Could you check a few things on this model? Use its own coordinates, in mm. Coordinates: 2 decimals unless noted, no trailing zeros. Write each loop counter-clockwise with the first axis right and the second up, starting at its lowest first coordinate (ties: lowest second). Pieces come first, ordered by that corner, then holes. Notation, with made-up numbers: (78, -20) - (92, -20) arc R15 cw to (92, -4) - close; hole circle Ø10 at (46, -11). An arc over 180 degrees is marked (long way). Write item = value, one per line. Start each with the question number.
```python
from build123d import *

# Parameters (mm, degrees)
F0_R     = 40
F1_DEPTH = 20
F2_R     = 5.08
F3_R     = 5.08


with BuildPart() as f1:
    # F0 (on Top) → F1 (new body)
    with BuildSketch(Plane.XY):
        with BuildLine():
            ThreePointArc((-115.457179, 96.407526), (-144.891009, 9.736149), (-61.108229, 46.597019))
            ThreePointArc((-61.108229, 46.597019), (-74.039839, 80.151967), (-106.145609, 96.350133))
            ThreePointArc((-106.145609, 96.350133), (-110.828783, 91.935219), (-115.457179, 96.407526))
        make_face()
        with Locations((-111.108229, 46.597019)):
            Circle(F0_R, mode=Mode.SUBTRACT)
    extrude(amount=F1_DEPTH)

    # F2
    f2_edges = [f1.edges().sort_by_distance(p)[0] for p in [
        (-151.108229, 46.597019, 20),
    ]]
    fillet(f2_edges, radius=F2_R)

    # F3
    f3_edges = [f1.edges().sort_by_distance(p)[0] for p in [
        (-151.108229, 46.597019, 0),
    ]]
    fillet(f3_edges, radius=F3_R)


solid = f1.part
```
1) If I drill on probe 1 along X at (y, z) = (22.5, 11); probe 2 along X at (y, z) = (50.5, 5.75); probe 3 along Y at (x, z) = (-92, 13.75), over which ranges is the centre line in solid material (lowest first)? Write a range as [from, to].
2) Suppose I cut it at B-B on z = 3.75. Please give me the cut outline in (x, y), plus the area to 3 significant figures.
3) Thinking about a two-plate mould opening in X: for faces 1 (the flat face through (-156, 39, 20)), 2 (the cylindrical face through (-151.07, 48.36, 9.93)), 3 (the cylindrical face through (-110.729, 91.936, 9.86)), which applies, +X half, -X half, draft (parallel to the pull), parting line (faces both ways), or undercut?
4) Suppose I cut it at A-A on z = 8.75. Please give me the cut outline in (x, y), plus the area to 3 significant figures.
5) For P1, Ø5, axis at y = 53.5, z = 12, coming from the -X side; P2, Ø3, axis at x = -76.5, z = 7, coming from the +Y side; P3, Ø3, axis at y = 35, z = 16, coming from the -X side, each with a flat end and sliding along its axis, tell me the tip position at first contact or that it passes through.
Reply:
q1.probe_1 = [-154.92, -143.04], [-79.18, -67.3]
q1.probe_2 = [-160.96, -150.92], [-71.3, -61.26]
q1.probe_3 = [0.39, 11.46], [81.74, 92.8]
q2.outline = (-115.46, 96.41) arc R50 ccw (long way) to (-61.11, 46.6) arc R50 ccw to (-106.15, 96.35) arc R4.66 cw to start; hole circle Ø80.35 at (-111.11, 46.6)
q2.area = 2,750 mm^2
q3.face_1 = draft
q3.face_2 = undercut
q3.face_3 = undercut
q4.outline = (-115.46, 96.41) arc R50 ccw (long way) to (-61.11, 46.6) arc R50 ccw to (-106.15, 96.35) arc R4.66 cw to start; hole circle Ø80 at (-111.11, 46.6)
q4.area = 2,790 mm^2
q5.P1 = -160.91
q5.P2 = 84.06
q5.P3 = -160.08
